Geometry: final body of the model. Coordinates: model frame, mm. A direction names the side the tool comes from. Give positions to 0.01 mm unless a question says otherwise; leave off trailing zeros. Loops run counter-clockwise (first coordinate to the right, second up) from the corner with the lowest first, then second, coordinate; pieces in that order, holes last. Notation, with made-up numbers: (-15.75, 1.5) -> (25.25, 1.5) arc R28 cw to (25.25, 25.5) -> close; hole circle Ø10 at (45.25, 48.25). An arc over 180 degrees is marked (long way). One line per item, written item: value. Start each with the question number.
from build123d import *

# Parameters (mm, degrees)
SKETCH1_W           = 203.2
SKETCH1_H           = 50.8
BOSS_EXTRUDE1_DEPTH = 3.175
SKETCH2_R           = 1.5
SKETCH2_W           = 45.6
SKETCH2_H           = 33.96
CUT_EXTRUDE1_DEPTH  = 3.175
SKETCH3_W           = 25.4
SKETCH3_H           = 3.175
BOSS_EXTRUDE2_DEPTH = 3.175


with BuildPart() as part:
    # Sketch1 → Boss-Extrude1 (new body)
    with BuildSketch(Plane.XY):
        Rectangle(SKETCH1_W, SKETCH1_H)
    extrude(amount=BOSS_EXTRUDE1_DEPTH)

    # Sketch2 → Cut-Extrude1 (cut)
    with BuildSketch(Plane.XY.offset(3.175)):
        with Locations((27.769072573, 17.082783056)):
            Circle(SKETCH2_R)
        with Locations((-28.364927427, 17.082783056)):
            Circle(SKETCH2_R)
        with Locations((-28.364927427, -16.699216944)):
            Circle(SKETCH2_R)
        with Locations((27.769072573, -16.699216944)):
            Circle(SKETCH2_R)
        Rectangle(SKETCH2_W, SKETCH2_H)
    extrude(amount=-CUT_EXTRUDE1_DEPTH, mode=Mode.SUBTRACT)

    # Sketch3 → Boss-Extrude2 (add)
    with BuildSketch(Plane.XY.offset(3.175)):
        with Locations((-38.1, 26.9875)):
            Rectangle(SKETCH3_W, SKETCH3_H)
        with Locations((-88.9, 26.9875)):
            Rectangle(SKETCH3_W, SKETCH3_H)
        with Locations((12.7, 26.9875)):
            Rectangle(SKETCH3_W, SKETCH3_H)
        with Locations((63.5, 26.9875)):
            Rectangle(SKETCH3_W, SKETCH3_H)
    extrude(amount=-BOSS_EXTRUDE2_DEPTH)


solid = part.part
Item 1: Section A-A, the plane y = -10.5. Output: boundary loops of the cut face in (x, z) (3 decimals), then the cut area to 3 significant figures.
Item 2: Mould query, pull axis X, two halves, no side actions, for faces 5 (the face through (76.2, 27, 2)), 6 (the face through (13, 28.575, 2)), 7 (the face through (-64, 25.4, 2)). Classes: pulls with the +X half, pulls with the -X half, needs draft (parallel to the pull), parting line crosses it, or undercut.
Item 3: Pin query (flat end, axial travel): pin 1 (1 mm diameter, centred on x = -15, z = 2.5, fed in from +Y); pin 2 (1.6 mm diameter, centred on y = 27.5, z = 1.5, fed in from +X). Return the tip coordinate at first contact, or that it passes through.
Item 4: Ray query, line 1 along Y through (x, z) = (27.5, 1.4); line 2 along X through (y, z) = (-15, 0.5); line 3 along Y through (x, z) = (11, 2.2) (3 decimals). Return the intervals inside material, ascending. Write a range as [from, to].
Item 5: Section D-D, the plane x = -60. Output: boundary loops of the cut face in (y, z) (3 decimals), then the cut area to 3 significant figures.
Item 6: Section C-C, the plane z = 1.1. Output: boundary loops of the cut face in (x, y) (3 decimals).
Item 7: Section B-B, the plane x = 18.5. Output: boundary loops of the cut face in (y, z) (3 decimals).
Item 8: Access query for faces 1 (the face through (38, 25.4, 2)), 2 (the face through (22.8, 0, 2)), 3 (the face through (89, 25.4, 2)), 4 (the face through (-1, -25.4, 2)). Directions: +Z, -Z, +X, -X, +Y, -Y. A direction counts if a zero-diameter tool reaches every point of the face in a straight line with its end or side. Return the directions, or none.
Geometry check:
1. outline: (-101.6, 0) -> (-22.8, 0) -> (-22.8, 3.175) -> (-101.6, 3.175) -> close; (22.8, 0) -> (101.6, 0) -> (101.6, 3.175) -> (22.8, 3.175) -> close
1. area: 500 mm2
2. face 5: pulls with the +X half
2. face 6: needs draft
2. face 7: undercut
3. pin 1: stops at y = 25.4
3. pin 2: stops at x = 76.2
4. line 1: y = [-25.4, -18.17], [-15.22, 15.61], [18.56, 25.4]
4. line 2: x = [-101.6, -22.8], [22.8, 101.6]
4. line 3: y = [-25.4, -16.98], [16.98, 28.575]
5. outline: (-25.4, 0) -> (25.4, 0) -> (25.4, 3.175) -> (-25.4, 3.175) -> close
5. area: 161 mm2
6. outline: (-101.6, -25.4) -> (101.6, -25.4) -> (101.6, 25.4) -> (76.2, 25.4) -> (76.2, 28.575) -> (50.8, 28.575) -> (50.8, 25.4) -> (25.4, 25.4) -> (25.4, 28.575) -> (0, 28.575) -> (0, 25.4) -> (-25.4, 25.4) -> (-25.4, 28.575) -> (-50.8, 28.575) -> (-50.8, 25.4) -> (-76.2, 25.4) -> (-76.2, 28.575) -> (-101.6, 28.575) -> close; hole circle Ø3 at (-28.365, -16.699); hole circle Ø3 at (-28.365, 17.083); hole (-22.8, -16.98) -> (22.8, -16.98) -> (22.8, 16.98) -> (-22.8, 16.98) -> close; hole circle Ø3 at (27.769, -16.699); hole circle Ø3 at (27.769, 17.083)
7. outline: (-25.4, 0) -> (-16.98, 0) -> (-16.98, 3.175) -> (-25.4, 3.175) -> close; (16.98, 0) -> (28.575, 0) -> (28.575, 3.175) -> (16.98, 3.175) -> close
8. face 1: +Z, -Z, +Y
8. face 2: +Z, -Z
8. face 3: +Z, -Z, +X, +Y
8. face 4: +Z, -Z, +X, -X, -Y
